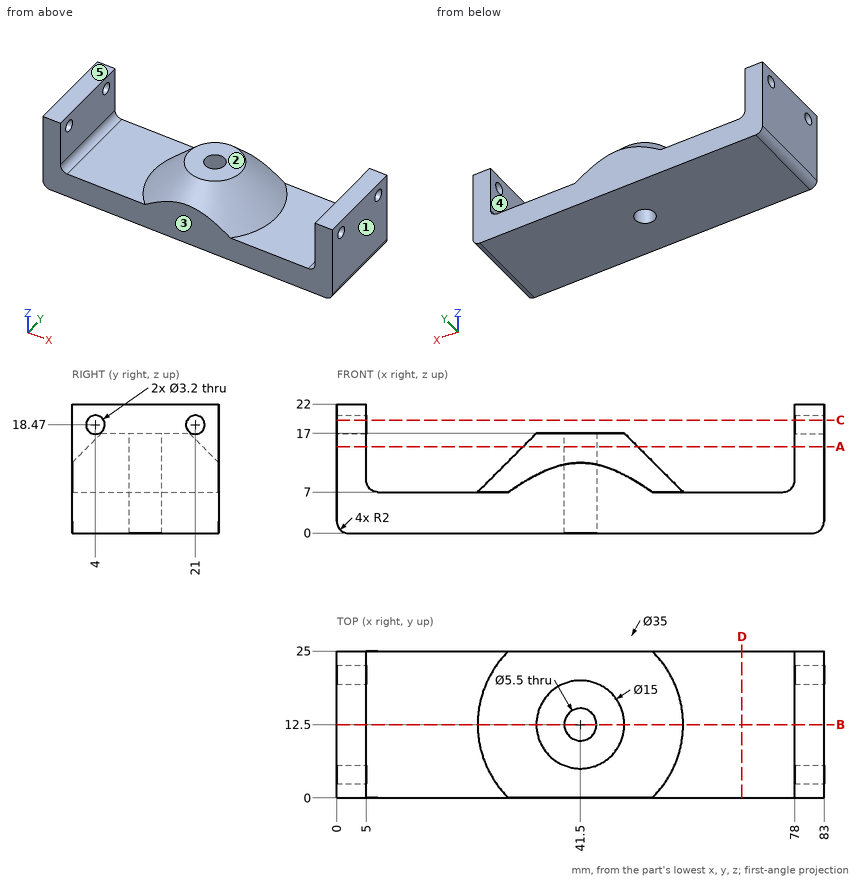
The drawing under review shows one solid part. Ordinate dimensions are in mm from its lowest x, y, z. A direction names the side the tool comes from. Round coordinates to 2 decimals unless told otherwise and drop trailing zeros. Loops run counter-clockwise (first coordinate to the right, second up) from the corner with the lowest first, then second, coordinate; pieces in that order, holes last. Notation, with made-up numbers: (-36.5, 61) - (-8.5, 61) arc R23 cw to (-8.5, 98) - close; hole circle Ø6 at (-11, 17). An arc over 180 degrees is marked (long way). One line per item, written item: value. Start each with the question number.
1) Insertion check: pin 1 Ø10 at (x, y) = (11.5, 5) entering from +Z; pin 2 Ø4.5 at (x, y) = (44, 10) entering from +Z; pin 3 Ø6.5 at (x, y) = (61, 14.5) entering from +Z. Each pin has a flat end and moves straight along its axis. Give the tip position at first contact, or say it passes through.
2) Consider section B-B on y = 12.5. Give the boundary of the cut face in (x, z).
3) Draft analysis for pull direction X (two halves, no side actions). For the marked faces 1, 2 and 3, state which applies: +X half, -X half, draft (parallel to the pull), parting line (faces both ways), or undercut.
4) Consider section A-A on z = 14.75. Give the boundary of the cut face in (x, y), then the cut area to 3 significant figures.
5) To check wall thickness, follow L1, parallel to X at y = 5, z = 21.25; L2, parallel to X at y = 14.5, z = 11.75; L3, parallel to X at y = 15, z = 6. State the ranges of each line that lie inside material, in increasing order. Write a range as from..to.
6) For the marked faces 4 and 5, list the 3-axis set-ups (+Z, -Z, +X, -X, +Y, -Y) from which the entire face can be reached by the end or side of a thin tool; tool diameter is ignored.
7) Consider section C-C on z = 19.25. Give the boundary of the cut face in (x, y).
8) Consider section D-D on x = 69. Give the boundary of the cut face in (y, z), then the cut area to 3 significant figures.
Reported:
1. pin 1: stops at z = 7.06
1. pin 2: stops at z = 17
1. pin 3: stops at z = 8.15
2. outline: (0, 2) arc R2 ccw to (2, 0) - (38.75, 0) - (38.75, 17) - (34, 17) - (24, 7) - (7, 7) arc R2 cw to (5, 9) - (5, 22) - (0, 22) - close; (44.25, 0) - (81, 0) arc R2 ccw to (83, 2) - (83, 22) - (78, 22) - (78, 9) arc R2 cw to (76, 7) - (59, 7) - (49, 17) - (44.25, 17) - close
3. face 1: +X half
3. face 2: undercut
3. face 3: draft
4. outline: (0, 0) - (5, 0) - (5, 25) - (0, 25) - close; circle Ø19.5 at (41.5, 12.5); (78, 0) - (83, 0) - (83, 25) - (78, 25) - close; hole circle Ø5.5 at (41.5, 12.5)
4. area: 525 mm^2
5. L1: x = 0..5, 78..83
5. L2: x = 0..5, 28.91..39.61, 43.39..54.09, 78..83
5. L3: x = 0..40.35, 42.65..83
6. face 4: +Z, +Y, -Y
6. face 5: +Z, +X, -X, +Y, -Y
7. outline: (0, 0) - (5, 0) - (5, 2.6) - (0, 2.6) - close; (0, 5.4) - (5, 5.4) - (5, 19.6) - (0, 19.6) - close; (0, 22.4) - (5, 22.4) - (5, 25) - (0, 25) - close; (78, 0) - (83, 0) - (83, 2.6) - (78, 2.6) - close; (78, 5.4) - (83, 5.4) - (83, 19.6) - (78, 19.6) - close; (78, 22.4) - (83, 22.4) - (83, 25) - (78, 25) - close
8. outline: (0, 0) - (25, 0) - (25, 7) - (0, 7) - close
8. area: 175 mm^2
